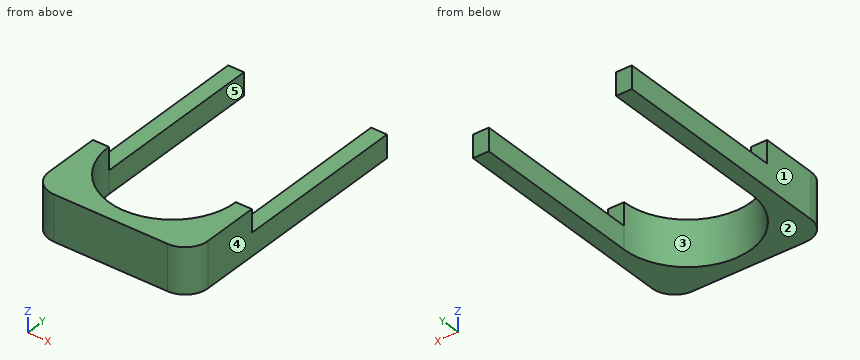
Autodesk Fusion 360 part; units mm, degrees
sketch "Sketch1" plane through (0, 0, 0) normal (0, 0, 1) x (1, 0, 0)
  circle A0 centre (0, 0) radius 14
  line L0 (14, 0) -> (-14, 0)
  line L1 (-17.5, 0) -> (-17.5, -17.5)
  line L2 (-17.5, -17.5) -> (17.5, -17.5)
  line L3 (17.5, -17.5) -> (17.5, 0)
  line L4 (-17.5, 0) -> (-17.5, 38.5)
  line L5 (17.5, 0) -> (17.5, 38.5)
  line L6 (-17.5, 0) -> (-17.5, 38.5)
  line L7 (-17.5, 38.5) -> (-14, 38.5)
  line L8 (-14, 38.5) -> (-14, 0)
  line L9 (17.5, 0) -> (17.5, 38.5)
  line L10 (17.5, 38.5) -> (14, 38.5)
  line L11 (14, 38.5) -> (14, 0)
  line L12 (-14, 38.5) -> (14, 38.5)
  arc A1 (-17.5, 0.003) -> (-17.5, -0.003) centre (0, 0) ccw
  line L13 (-17.5, 0) -> (-14, 0)
  line L14 (17.5, 0) -> (14, 0)
  dimension "d1" = 28
  dimension "d2" = 35
  dimension "d3" = 35
  dimension "d4" = 17.5
  dimension "d5" = 38.5
  dimension "d6" = 38.5
extrude "Extrude1" add sketch "Sketch1" along normal blind 10 contours A0 L1 L2 L3 A1 L13 L14
extrude "Extrude2" add sketch "Sketch1" along normal blind 5 contours L5 L9 L10 L11 L14 | L4 L6 L7 L8 A1 L13
fillet "Fillet1" radius 5 2 edges at (-17.5, -17.5, 5) (17.5, -17.5, 5)
The model under review builds one solid part; all positions refer to its coordinate system, in mm. Face numbers are marked on the shaded views. A direction names the side the tool comes from. Round coordinates to 2 decimals unless told otherwise and drop trailing zeros. Order: outer loops, then holes, each group sorted by start corner. A loop starts at its lowest first (then second) coordinate and runs counter-clockwise, first axis right, second up. Notation, with made-up numbers: (-28, 60.25) - (-5, 60.25) arc R34 cw to (-5, 94.25) - close; hole circle Ø9 at (33.5, 89). An arc over 180 degrees is marked (long way). Use one line per item in the form item = value.
Q1. Clearance check with flat-ended pins moving along their axes: P1, Ø1, axis at x = -9.5, z = 7, coming from the +Y side; P2, Ø3, axis at x = -16.5, y = 25.5, coming from the +Z side; P3, Ø3, axis at x = -16.5, z = 8.5, coming from the +Y side. State where each tip first meets the part, or that it passes through.
Response values:
P1 = -9.8
P2 = 5
P3 = 0
Q2. Add section A-A on y = 1.5. Give the boundary of the cut face in (x, z).
Response values:
outline = (-17.5, 0) - (-14, 0) - (-14, 5) - (-17.5, 5) - close; (14, 0) - (17.5, 0) - (17.5, 5) - (14, 5) - close
Q3. Tool access review of the marked faces 4 and 5: name each direction out of +Z, -Z, +X, -X, +Y, -Y from which nothing blocks a thin tool from reaching the whole face with its end or side.
Response values:
face_4 = +Z, -Z, +X, +Y, -Y
face_5 = +Z, -Z, +Y
Q4. Mouldability with a two-part tool opening along X and no side actions: class the marked faces 1, 2 and 3 as pulls with the +X half, pulls with the -X half, needs draft (parallel to the pull), parting line crosses it, or undercut.
Response values:
face_1 = pulls with the -X half
face_2 = needs draft
face_3 = undercut
Q5. Add section B-B on z = 3. Give the boundary of the cut face in (x, y), then the cut area to 3 significant figures.
Response values:
outline = (-17.5, -12.5) arc R5 ccw to (-12.5, -17.5) - (12.5, -17.5) arc R5 ccw to (17.5, -12.5) - (17.5, 38.5) - (14, 38.5) - (14, 0) arc R14 cw to (-14, 0) - (-14, 38.5) - (-17.5, 38.5) - close
area = 563 mm^2
Q6. Add section D-D on z = 7.5. Give the boundary of the cut face in (x, y).
Response values:
outline = (-17.5, -12.5) arc R5 ccw to (-12.5, -17.5) - (12.5, -17.5) arc R5 ccw to (17.5, -12.5) - (17.5, 0) - (14, 0) arc R14 cw to (-14, 0) - (-17.5, 0) - close
Q7. To check wall thickness, follow line 1 (X direction, y = 4, z = 4.25); line 2 (X direction, y = -2, z = 8); line 3 (Y direction, x = -0.5, z = 1.75). State the ranges of each line that lie inside material, in increasing order.
Response values:
line_1 = -17.5 to -14, 14 to 17.5
line_2 = -17.5 to -13.86, 13.86 to 17.5
line_3 = -17.5 to -13.99
Q8. Add section C-C on x = -15. Give the boundary of the cut face in (y, z), then the cut area to 3 significant figures.
Response values:
outline = (-16.83, 0) - (38.5, 0) - (38.5, 5) - (0, 5) - (0, 10) - (-16.83, 10) - close
area = 361 mm^2
